Check sheet for the modelled part. Datum: model origin and axes. Units: mm. Face numbers are marked on the shaded views. A direction names the side the tool comes from. Round coordinates to 2 decimals unless told otherwise and drop trailing zeros. Write each loop counter-clockwise with the first axis right and the second up, starting at its lowest first coordinate (ties: lowest second). Pieces come first, ordered by that corner, then holes.
Item 1: Release check for a two-part mould opening along X. For the marked faces 4, 5, 6 and 7 record: +X half, -X half, draft (parallel to the pull), parting line (faces both ways), or undercut.
Item 2: Go/stop test with flat-tipped pins: pin 1 Ø1.3 at (y, z) = (39, 18) entering from +X; pin 2 Ø10 at (y, z) = (11, 4) entering from +X; pin 3 Ø0.7 at (y, z) = (38.5, 19) entering from -X. Record where each tip stops, or that it passes through.
Item 3: Material ranges on line 1 (X direction, y = 22, z = 8.5); line 2 (X direction, y = 30, z = 10.25); line 3 (X direction, y = 15.5, z = 14.5), recorded low to high.
Item 4: Tool access check on the marked faces 1, 2 and 3. Record the directions out of +Z, -Z, +X, -X, +Y, -Y that give a thin tool (end or side, any length) a straight path to the whole face; none if there is none.
Item 5: Cross-section at C-C on z = 17. Enter the section's corners in (x, y).
Item 6: Cross-section at D-D on x = -10.5. Enter the section's corners in (y, z).
Item 7: Cross-section at B-B on y = 19. Count the separate pieces of the cut face and the enclosed holes in it, plus the area to 3 significant figures.
Item 8: Cross-section at A-A on x = 9. Enter the section's corners in (y, z), plus the area to 3 significant figures.
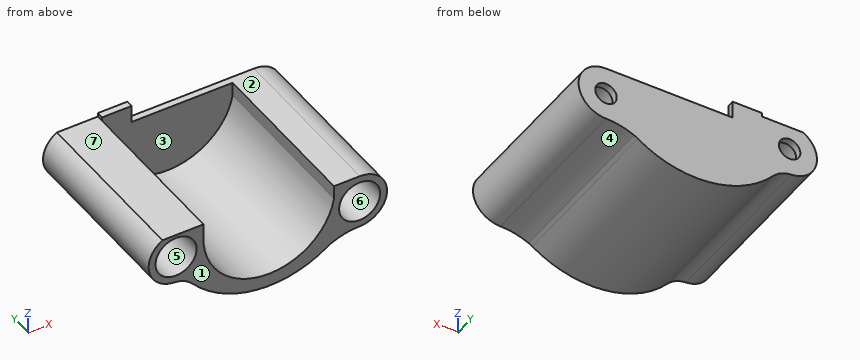
from build123d import *

# Parameters (mm, degrees)
SKETCH2_R           = 4.7625
BOSS_EXTRUDE1_DEPTH = 38.1
SKETCH3_R           = 2.4892
BOSS_EXTRUDE2_DEPTH = 1.5875
SKETCH4_W           = 6.858
SKETCH4_H           = 4.056568305
SKETCH4_W_2         = 20.112893425
SKETCH4_H_2         = 3.175
BOSS_EXTRUDE3_DEPTH = 1.5875
FILLET2_R           = 6.35


with BuildPart() as part:
    # Sketch2 → Boss-Extrude1 (new body)
    with BuildSketch(Plane(origin=(0, 0, 0), x_dir=(1, 0, 0), z_dir=(0, 1, 0))):
        with BuildLine():
            Line((-13.637822674, -18.9154966), (-13.637822674, -15.7404966))
            ThreePointArc((-13.637822674, -15.7404966), (0, 0), (16.609085938, -12.5654966))
            Line((16.609085938, -12.5654966), (16.609085938, -15.7404966))
            Line((16.609085938, -15.7404966), (22.545691393, -15.7404966))
            ThreePointArc((22.545691393, -15.7404966), (28.895691393, -9.3904966), (22.545691393, -3.0404966))
            ThreePointArc((22.545691393, -3.0404966), (18.914562129, -2.601594541), (15.492581173, -1.310168551))
            ThreePointArc((15.492581173, -1.310168551), (-2.207478742, 2.815047226), (-17.640279185, -6.783817119))
            ThreePointArc((-17.640279185, -6.783817119), (-18.810770101, -6.984553123), (-19.996688426, -7.047335697))
            ThreePointArc((-19.996688426, -7.047335697), (-26.135207048, -11.772192893), (-23.138726022, -18.9154966))
            Line((-23.138726022, -18.9154966), (-13.637822674, -18.9154966))
        make_face()
        with Locations((-19.996688426, -13.397335697)):
            Circle(SKETCH2_R, mode=Mode.SUBTRACT)
        with Locations((22.545691393, -9.3904966)):
            Circle(SKETCH2_R, mode=Mode.SUBTRACT)
    extrude(amount=BOSS_EXTRUDE1_DEPTH)

    # Sketch3 → Boss-Extrude2 (add)
    with BuildSketch(Plane(origin=(0, 38.1, 0), x_dir=(-1, 0, 0), z_dir=(0, 1, 0))):
        with BuildLine():
            Line((13.637822674, 15.7404966), (3.503807487, 15.7404966))
            Line((3.503807487, 15.7404966), (3.503807487, 12.5654966))
            Line((3.503807487, 12.5654966), (-16.609085938, 12.5654966))
            Line((-16.609085938, 12.5654966), (-16.609085938, 15.7404966))
            Line((-16.609085938, 15.7404966), (-22.545691393, 15.7404966))
            ThreePointArc((-22.545691393, 15.7404966), (-28.895691393, 9.3904966), (-22.545691393, 3.0404966))
            ThreePointArc((-22.545691393, 3.0404966), (-18.914562129, 2.601594541), (-15.492581173, 1.310168551))
            ThreePointArc((-15.492581173, 1.310168551), (2.207478742, -2.815047226), (17.640279185, 6.783817119))
            ThreePointArc((17.640279185, 6.783817119), (18.810770101, 6.984553123), (19.996688426, 7.047335697))
            ThreePointArc((19.996688426, 7.047335697), (26.135207048, 11.772192893), (23.138726022, 18.9154966))
            Line((23.138726022, 18.9154966), (13.637822674, 18.9154966))
            Line((13.637822674, 18.9154966), (13.637822674, 15.7404966))
        make_face()
        with Locations((-22.545691393, 9.3904966)):
            Circle(SKETCH3_R, mode=Mode.SUBTRACT)
        with Locations((19.996688426, 13.397335697)):
            Circle(SKETCH3_R, mode=Mode.SUBTRACT)
    extrude(amount=BOSS_EXTRUDE2_DEPTH)

    # Sketch4 → Boss-Extrude3 (add)
    with BuildSketch(Plane(origin=(0, 39.6875, 0), x_dir=(-1, 0, 0), z_dir=(0, 1, 0))):
        with Locations((10.208822674, 17.768780752)):
            Rectangle(SKETCH4_W, SKETCH4_H)
        with Locations((-6.552639226, 14.1529966)):
            Rectangle(SKETCH4_W_2, SKETCH4_H_2)
    extrude(amount=-BOSS_EXTRUDE3_DEPTH)

    # Fillet2
    fillet2_edges = [part.edges().sort_by_distance(p)[0] for p in [
        (15.492581173, 19.84375, 1.310168551),
        (-17.640279185, 19.84375, 6.783817119),
    ]]
    fillet(fillet2_edges, radius=FILLET2_R)


solid = part.part
Response values:
1. face 4: +X half
1. face 5: undercut
1. face 6: undercut
1. face 7: draft
2. pin 1: stops at x = -6.78
2. pin 2: stops at x = 28.88
2. pin 3: stops at x = -23.56
3. line 1: x = -24.04 to -12.12, 15.3 to 17.87, 27.22 to 28.83
3. line 2: x = -25.51 to -23.57, -16.42 to -12.84, 16.02 to 17.86, 27.23 to 28.84
3. line 3: x = -26.25 to -24.63, -15.36 to -13.63, 16.61 to 26.32
4. face 1: +Z, -Z, +X, -X, -Y
4. face 2: +Z, +X, +Y, -Y
4. face 3: +Z, -Y
5. outline: (-25.23, 0) - (-23.11, 0) - (-23.11, 38.1) - (-16.88, 38.1) - (-16.88, 0) - (-13.64, 0) - (-13.64, 38.1) - (-6.78, 38.1) - (-6.78, 39.69) - (-25.23, 39.69) - close
6. outline: (0, 0.22) - (39.69, 0.22) - (39.69, 19.8) - (38.1, 19.8) - (38.1, 5.88) - (0, 5.88) - close
7. separate pieces: 1
7. enclosed holes: 2
7. area: 284 mm2
8. outline: (0, -1.97) - (39.69, -1.97) - (39.69, 15.74) - (38.1, 15.74) - (38.1, 1.84) - (0, 1.84) - close
8. area: 173 mm2
